Can you work these out from the model? Positions are in its coordinate system, mm. A direction names the side the tool comes from. Coordinates: 2 decimals unless noted, no trailing zeros. Order: outer loops, then holes, each group sorted by start corner. A loop starts at its lowest first (then second) coordinate and runs counter-clockwise, first axis right, second up. Notation, with made-up numbers: (-38, 69) -> (7, 69) arc R21 ccw to (7, 96) -> close; hole circle Ø1 at (22, 13). An arc over 180 degrees is marked (long way). Answer in a Markdown table with one row per item. Add a question column.
1. Will these pins go through, and if not, where does the flat tip stop? pin 1 (2.5 mm diameter, centred on x = -2.5, y = 3.5, fed in from -Z); pin 2 (2.5 mm diameter, centred on y = 5, z = -8, fed in from -X); pin 3 (1.5 mm diameter, centred on x = -0.5, z = 5.5, fed in from +Y); pin 4 (12 mm diameter, centred on y = 16.5, z = 2, fed in from -X).
2. Imagine slicing it at C-C on z = 7. Write out the boundary of the cut face in (x, y).
3. Imagine slicing it at A-A on y = 12.5. Write out the boundary of the cut face in (x, z), plus the area to 3 significant figures.
4. On a 3-axis mill with a long thin cutter (end or side, diameter ignored), from which of +Z, -Z, +X, -X, +Y, -Y can I reach the whole of each face in a straight line? I mean faces 1 (the face through (-3, -38.004, 0)), 2 (the face through (-1.715, 0, -8)), 3 (the face through (-1.715, 0, 7)). Say none if no direction works.
5. If I drill on line 1 along Y through (x, z) = (-1, -5.75); line 2 along Z through (x, y) = (-2, -20.5); line 3 along Y through (x, z) = (0.75, -0.25), over which ranges is the centre line in solid material (lowest first)? Write a range as [from, to].
6. Imagine slicing it at B-B on x = -3. Write out the boundary of the cut face in (y, z).
7. We'd pull the mould along Z, two halves only. Please class faces 4 (the face through (-2.195, -2.985, 0.014)), 5 (the face through (-1, -1, 9.027)), 6 (the face through (0, 3, 10)): pulls with the +Z half, pulls with the -Z half, needs draft (parallel to the pull), parting line crosses it, or undercut.
from build123d import *

# Parameters (mm, degrees)
SKETCH1_W               = 23.666666666
SKETCH1_H               = 86
BOSS_EXTRUDE1_DEPTH     = 3
SKETCH2_W               = 5
SKETCH2_H               = 3
CUT_EXTRUDE1_DEPTH      = 45.699303997
SKETCH3_W               = 18.054262684
SKETCH3_H               = 80.34146894
BOSS_EXTRUDE2_DEPTH     = 5
SKETCH5_W               = 11.91581337
SKETCH5_H               = 76.008445896
CUT_EXTRUDE2_DEPTH      = 5
CUT_EXTRUDE3_DEPTH      = 45.877920827
CUT_EXTRUDE3_DEPTH_BACK = 45.877920827
SKETCH7_W               = 2
SKETCH7_H               = 9
BOSS_EXTRUDE3_DEPTH     = 5
CUT_EXTRUDE4_DEPTH      = 5
SKETCH9_W               = 2.534423144
SKETCH9_H               = 2
CUT_EXTRUDE5_DEPTH      = 1
CUT_EXTRUDE6_DEPTH      = 2
BOSS_EXTRUDE5_DEPTH     = 2
BOSS_EXTRUDE6_DEPTH     = 2
CUT_EXTRUDE7_START      = -2
CUT_EXTRUDE7_DEPTH      = 2


with BuildPart() as part:
    # Sketch1 → Boss-Extrude1 (new body)
    with BuildSketch(Plane(origin=(0, 0, 0), x_dir=(0, 0, -1), z_dir=(1, 0, 0))):
        Rectangle(SKETCH1_W, SKETCH1_H)
    extrude(amount=BOSS_EXTRUDE1_DEPTH)

    # Sketch2 → Cut-Extrude1 (cut, through all)
    with BuildSketch(Plane(origin=(3, 0, 0), x_dir=(0, 0, -1), z_dir=(1, 0, 0))):
        with Locations((0, -34.060962647)):
            Rectangle(SKETCH2_W, SKETCH2_H)
    extrude(amount=-CUT_EXTRUDE1_DEPTH, mode=Mode.SUBTRACT)

    # Sketch3 → Boss-Extrude2 (add)
    with BuildSketch(Plane.ZY):
        Rectangle(SKETCH3_W, SKETCH3_H)
    extrude(amount=BOSS_EXTRUDE2_DEPTH)

    # Sketch5 → Cut-Extrude2 (cut)
    with BuildSketch(Plane.ZY.offset(5)):
        Rectangle(SKETCH5_W, SKETCH5_H)
    extrude(amount=-CUT_EXTRUDE2_DEPTH, mode=Mode.SUBTRACT)

    # Sketch6 → Cut-Extrude3 (cut, two sides: drawn at the far end of the back side and taken through both)
    with BuildSketch(Plane.XY.offset(-CUT_EXTRUDE3_DEPTH_BACK)):
        Polygon((-5, -19.974207963), (-1.714874455, -16.689082418), (-1.714874455, 16.689082418), (-5, 19.974207963), align=None)
    extrude(amount=CUT_EXTRUDE3_DEPTH + CUT_EXTRUDE3_DEPTH_BACK, mode=Mode.SUBTRACT)

    # Sketch7 → Boss-Extrude3 (add)
    with BuildSketch(Plane.ZY):
        Rectangle(SKETCH7_W, SKETCH7_H)
    extrude(amount=BOSS_EXTRUDE3_DEPTH)

    # Sketch8 → Cut-Extrude4 (cut)
    with BuildSketch(Plane.XY.offset(1)):
        with BuildLine():
            ThreePointArc((-5, -0.459578833), (-2.44210099, -2.530530169), (0, -0.32421434))
            Line((0, -0.32421434), (0, 0.32421434))
            ThreePointArc((0, 0.32421434), (-2.44210099, 2.530530169), (-5, 0.459578833))
            Line((-5, 0.459578833), (-5, -0.459578833))
        make_face()
        with BuildLine():
            Line((-5, -4.5), (-2.510609776, -4.5))
            ThreePointArc((-2.510609776, -4.5), (-3.81075192, -4.308088951), (-5, -3.748724625))
            Line((-5, -3.748724625), (-5, -4.5))
        make_face()
        with BuildLine():
            Line((-2.510609776, -4.5), (0, -4.5))
            Line((0, -4.5), (0, -3.734546632))
            ThreePointArc((0, -3.734546632), (-1.198256898, -4.304384965), (-2.510609776, -4.5))
        make_face()
        with BuildLine():
            ThreePointArc((-2.510609794, 4.5), (-1.198256907, 4.304384967), (0, 3.734546632))
            Line((0, 3.734546632), (0, 4.5))
            Line((0, 4.5), (-2.510609794, 4.5))
        make_face()
        with BuildLine():
            ThreePointArc((-5, 3.748724625), (-3.810751929, 4.308088948), (-2.510609794, 4.5))
            Line((-2.510609794, 4.5), (-5, 4.5))
            Line((-5, 4.5), (-5, 3.748724625))
        make_face()
    extrude(amount=-CUT_EXTRUDE4_DEPTH, mode=Mode.SUBTRACT)

    # Sketch9 → Cut-Extrude5 (cut)
    with BuildSketch(Plane.ZY.offset(5)):
        Rectangle(SKETCH9_W, SKETCH9_H)
    extrude(amount=-CUT_EXTRUDE5_DEPTH, mode=Mode.SUBTRACT)

    # Sketch12 → Cut-Extrude6 (cut)
    with BuildSketch(Plane.XY.offset(1)):
        with BuildLine():
            Line((-4.836179898, -1), (-5, -1))
            Line((-5, -1), (-5, -3.748724625))
            ThreePointArc((-5, -3.748724625), (-2.497849634, -4.499981909), (0, -3.734546632))
            Line((0, -3.734546632), (0, -0.32421434))
            ThreePointArc((0, -0.32421434), (-2.160279243, -2.507098902), (-4.836179898, -1))
        make_face()
        with BuildLine():
            Line((-5, 3.748724625), (-5, 1))
            Line((-5, 1), (-4.836179898, 1))
            ThreePointArc((-4.836179898, 1), (-2.160279243, 2.507098902), (0, 0.32421434))
            Line((0, 0.32421434), (0, 3.734546632))
            ThreePointArc((0, 3.734546632), (-2.497849634, 4.499981909), (-5, 3.748724625))
        make_face()
    extrude(amount=-CUT_EXTRUDE6_DEPTH, mode=Mode.SUBTRACT)

    # Sketch10 → Boss-Extrude5 (add)
    with BuildSketch(Plane.XY.offset(1)):
        with BuildLine():
            Line((0.632034053, -1.144834058), (-0.193, -4.453864907))
            ThreePointArc((-0.193, -4.453864907), (-2.801828378, -4.592278965), (-5.047908598, -3.258012274))
            Line((-5.047908598, -3.258012274), (-4.41989103, -0.739171385))
            Line((-4.41989103, -0.739171385), (-4.335953587, -0.66680401))
            ThreePointArc((-4.335953587, -0.66680401), (-2.053682052, -3.002243354), (0.632034053, -1.144834058))
        make_face()
        with BuildLine():
            Line((-5.047908598, 3.258012274), (-4.41989103, 0.739171385))
            Line((-4.41989103, 0.739171385), (-4.335953587, 0.66680401))
            ThreePointArc((-4.335953587, 0.66680401), (-2.053682052, 3.002243354), (0.632034053, 1.144834058))
            Line((0.632034053, 1.144834058), (-0.193, 4.453864907))
            ThreePointArc((-0.193, 4.453864907), (-2.801828378, 4.592278965), (-5.047908598, 3.258012274))
        make_face()
    extrude(amount=-BOSS_EXTRUDE5_DEPTH)

    # Sketch13 → Boss-Extrude6 (add)
    with BuildSketch(Plane(origin=(0, 0, -1), x_dir=(-1, 0, 0), z_dir=(0, 0, -1))):
        Polygon((0, 3.679784186), (0.193, 4.453864907), (-0.617433114, 4.244828064), (-0.739085506, -4.079345447), (0.193, -4.453864907), (0, -3.679784186), (0, -2.250971384), (0, 2.250971384), align=None)
    extrude(amount=-BOSS_EXTRUDE6_DEPTH)

    # Sketch15 → Cut-Extrude7 (cut)
    with BuildSketch(Plane(origin=(0, 0, -1), x_dir=(-1, 0, 0), z_dir=(0, 0, -1)).offset(CUT_EXTRUDE7_START)):
        Polygon((4.65583066, 1.685473556), (5.047908598, 3.258012274), (4.038538563, 1.685473556), align=None)
        with BuildLine():
            Line((4.65583066, 1.685473556), (4.038538563, 1.685473556))
            ThreePointArc((4.038538563, 1.685473556), (4.241224486, 1.191898546), (4.335953587, 0.66680401))
            Line((4.335953587, 0.66680401), (4.41989103, 0.739171385))
            Line((4.41989103, 0.739171385), (4.65583066, 1.685473556))
        make_face()
        with BuildLine():
            ThreePointArc((4.335953587, -0.66680401), (4.241224486, -1.191898546), (4.038538563, -1.685473556))
            Line((4.038538563, -1.685473556), (4.65583066, -1.685473556))
            Line((4.65583066, -1.685473556), (4.41989103, -0.739171385))
            Line((4.41989103, -0.739171385), (4.335953587, -0.66680401))
        make_face()
        Polygon((4.65583066, -1.685473556), (4.038538563, -1.685473556), (5.047908598, -3.258012274), align=None)
    extrude(amount=CUT_EXTRUDE7_DEPTH, mode=Mode.SUBTRACT)


solid = part.part
Answers follow:
| question | item | result |
|---|---|---|
| 1 | pin 1 | stops at z = -9.03 |
| 1 | pin 2 | stops at x = -1.71 |
| 1 | pin 3 | stops at y = 43 |
| 1 | pin 4 | stops at x = -5 |
| 2 | outline | (-5, -40.17) -> (0, -40.17) -> (0, -43) -> (3, -43) -> (3, 43) -> (0, 43) -> (0, 40.17) -> (-5, 40.17) -> (-5, 19.97) -> (-1.71, 16.69) -> (-1.71, -16.69) -> (-5, -19.97) -> close |
| 3 | outline | (-1.71, -9.03) -> (0, -9.03) -> (0, -11.83) -> (3, -11.83) -> (3, 11.83) -> (0, 11.83) -> (0, 9.03) -> (-1.71, 9.03) -> (-1.71, 5.96) -> (0, 5.96) -> (0, -5.96) -> (-1.71, -5.96) -> close |
| 3 | area | 81.5 mm² |
| 4 | face 1 | -X |
| 4 | face 2 | -Z, -X |
| 4 | face 3 | +Z, -X |
| 5 | line 1 | y = [-40.17, -38], [38, 40.17] |
| 5 | line 2 | z = [-9.03, -5.96], [5.96, 9.03] |
| 5 | line 3 | y = [-43, -35.56], [-32.56, 43] |
| 6 | outline | (-40.17, -9.03) -> (-17.97, -9.03) -> (-17.97, -5.96) -> (-38, -5.96) -> (-38, 5.96) -> (-17.97, 5.96) -> (-17.97, 9.03) -> (-40.17, 9.03) -> close; (-4.54, -1) -> (-2.72, -1) -> (-2.72, 1) -> (-4.54, 1) -> close; (2.72, -1) -> (4.54, -1) -> (4.54, 1) -> (2.72, 1) -> close; (17.97, -9.03) -> (40.17, -9.03) -> (40.17, 9.03) -> (17.97, 9.03) -> (17.97, 5.96) -> (38, 5.96) -> (38, -5.96) -> (17.97, -5.96) -> close |
| 7 | face 4 | undercut |
| 7 | face 5 | pulls with the +Z half |
| 7 | face 6 | needs draft |
